Model file for the job. Use its own axes, mm. A direction names the side the tool comes from. Round coordinates to 2 decimals unless told otherwise and drop trailing zeros. Order: outer loops, then holes, each group sorted by start corner. A loop starts at its lowest first (then second) coordinate and runs counter-clockwise, first axis right, second up. Notation, with made-up numbers: M -9.5,61 L 33.5,61 A30 ccw 33.5,91 Z; hole C 51.25,-24 d4. An arc over 180 degrees is marked long. Return JSON: item names as keys, results as strings. Group by question number.
Item 1: Which spindle directions (+Z, -Z, +X, -X, +Y, -Y) get a long thin tool onto all of the face, cutting with end or side? Do faces 4 (the face through (-30.48, 0, 8)), 5 (the face through (27.588, 0.689, 10.525)). Say none if no direction does.
Item 2: Pin check, flat tips, straight feed: pin 1 Ø4 at (x, y) = (25.4, 0) entering from -Z; pin 2 Ø3 at (x, y) = (-34.5, 1.5) entering from +Z. Stop position of each tip, or through.
Item 3: Slice it at A-A on z = 7. Write the cut outline in (x, y).
Item 4: Probe line 1 along X through (y, z) = (5.25, 10.5); line 2 along Y through (x, z) = (25.4, 7.75); line 3 along X through (y, z) = (1, 7.5). List the from-to ranges inside material, lowest first.
Item 5: Slice it at C-C on x = -25.4. Write the cut outline in (y, z), then the cut area to 3 significant figures.
Item 6: Slice it at D-D on z = 11.5. Write the cut outline in (x, y).
Item 7: Pull direction Y, two halves, no side cores. Call faces 1 (the face through (-1, 6.35, 2)), 2 (the face through (-1, -6.35, 2)), 3 (the face through (23.22, 0.1, 5.13)): pulls with the +Y half, pulls with the -Y half, needs draft (parallel to the pull), parting line crosses it, or undercut.
Item 8: Slice it at B-B on y = 0. Give the number of separate pieces and of enclosed holes in the cut face, then the cut area to 3 significant figures.
from build123d import *

# Parameters (mm, degrees)
SKETCH_W        = 88.9
SKETCH_H        = 12.7
SKETCH_R        = 2.182812
PAD_DEPTH       = 12.7
CHAMFER_SIZE    = 1
CHAMFER001_SIZE = 2.286
SKETCH001_W     = 10.16
SKETCH001_H     = 12.7
SKETCH001_W_2   = 40.64
POCKET_DEPTH    = 10.16
CHAMFER002_SIZE = 0.254


with BuildPart() as part:
    # Sketch → Pad (new body)
    with BuildSketch(Plane.XY):
        Rectangle(SKETCH_W, SKETCH_H)
        with Locations((-25.4, 0)):
            Circle(SKETCH_R, mode=Mode.SUBTRACT)
        with Locations((25.4, 0)):
            Circle(SKETCH_R, mode=Mode.SUBTRACT)
    extrude(amount=PAD_DEPTH)

    # Chamfer
    chamfer_edges = [part.edges().sort_by_distance(p)[0] for p in [
        (44.45, 6.35, 6.35),
        (44.45, -6.35, 6.35),
        (-44.45, -6.35, 6.35),
        (-44.45, 6.35, 6.35),
    ]]
    chamfer(chamfer_edges, length=CHAMFER_SIZE)

    # Chamfer001
    chamfer001_edges = [part.edges().sort_by_distance(p)[0] for p in [
        (-27.582812, 0, 12.7),
        (23.217187, 0, 12.7),
    ]]
    chamfer(chamfer001_edges, length=CHAMFER001_SIZE)

    # Sketch001 → Pocket (cut)
    with BuildSketch(Plane.XY.offset(12.7)):
        with Locations((-35.56, 0)):
            Rectangle(SKETCH001_W, SKETCH001_H)
        with Locations((35.56, 0)):
            Rectangle(SKETCH001_W, SKETCH001_H)
        Rectangle(SKETCH001_W_2, SKETCH001_H)
    extrude(amount=-POCKET_DEPTH, mode=Mode.SUBTRACT)

    # Chamfer002
    chamfer002_edges = [part.edges().sort_by_distance(p)[0] for p in [
        (-40.64, 0, 12.7),
        (-30.48, 0, 12.7),
        (-20.32, 0, 12.7),
        (20.32, 0, 12.7),
        (30.48, 0, 12.7),
        (40.64, 0, 12.7),
    ]]
    chamfer(chamfer002_edges, length=CHAMFER002_SIZE)


solid = part.part
Output values:
{
 "1": {"face 4": "+Z, +Y, -Y", "face 5": "+Z"},
 "2": {"pin 1": "through", "pin 2": "z = 2.54"},
 "3": {"outline": "M -44.45,-5.35 L -43.45,-6.35 L -40.64,-6.35 L -40.64,6.35 L -43.45,6.35 L -44.45,5.35 Z; M -30.48,-6.35 L -20.32,-6.35 L -20.32,6.35 L -30.48,6.35 Z; M 20.32,-6.35 L 30.48,-6.35 L 30.48,6.35 L 20.32,6.35 Z; M 40.64,-6.35 L 43.45,-6.35 L 44.45,-5.35 L 44.45,5.35 L 43.45,6.35 L 40.64,6.35 Z; hole C -25.4,0 d4.37; hole C 25.4,0 d4.37"},
 "4": {"line 1": "-44.45 to -40.64, -30.48 to -20.32, 20.32 to 30.48, 40.64 to 44.45", "line 2": "-6.35 to -2.18, 2.18 to 6.35", "line 3": "-44.45 to -40.64, -30.48 to -27.34, -23.46 to -20.32, 20.32 to 23.46, 27.34 to 30.48, 40.64 to 44.45"},
 "5": {"outline": "M -6.35,0 L -2.18,0 L -2.18,10.41 L -4.47,12.7 L -6.35,12.7 Z; M 2.18,0 L 6.35,0 L 6.35,12.7 L 4.47,12.7 L 2.18,10.41 Z", "area": "101 mm²"},
 "6": {"outline": "M -44.45,-5.35 L -43.45,-6.35 L -40.64,-6.35 L -40.64,6.35 L -43.45,6.35 L -44.45,5.35 Z; M -30.48,-6.35 L -20.32,-6.35 L -20.32,6.35 L -30.48,6.35 Z; M 20.32,-6.35 L 30.48,-6.35 L 30.48,6.35 L 20.32,6.35 Z; M 40.64,-6.35 L 43.45,-6.35 L 44.45,-5.35 L 44.45,5.35 L 43.45,6.35 L 40.64,6.35 Z; hole C -25.4,0 d6.54; hole C 25.4,0 d6.54"},
 "7": {"face 1": "pulls with the +Y half", "face 2": "pulls with the -Y half", "face 3": "undercut"},
 "8": {"separate pieces": "3", "enclosed holes": "0", "area": "388 mm²"}
}
